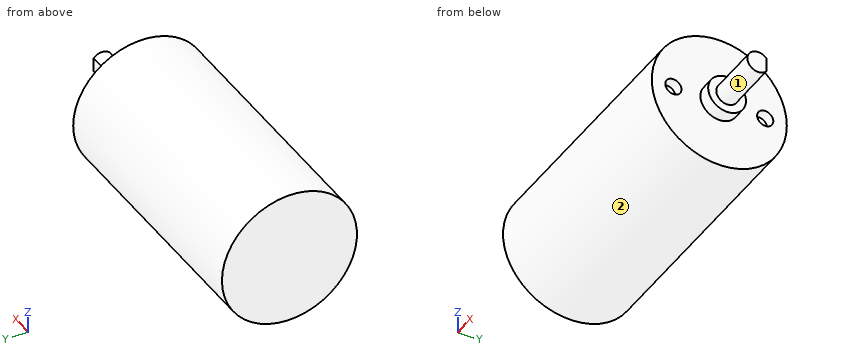
Autodesk Inventor part; units mm, degrees
ref_plane "YZ Plane" through (0, 0, 0) normal (1, 0, 0) x (0, 1, 0)
ref_plane "XZ Plane" through (0, 0, 0) normal (0, 1, 0) x (-1, 0, 0)
ref_plane "XY Plane" through (0, 0, 0) normal (0, 0, 1) x (1, 0, 0)
sketch "Sketch1" plane through (0, 0, 0) normal (1, 0, 0) x (0, 1, 0)
  circle A0 centre (0, 0) radius 12.5
  dimension "d0" = 25
extrude "Extrusion1" add sketch "Sketch1" along normal blind 47.8
sketch "Sketch2" plane through (47.8, 0, 0) normal (1, 0, 0) x (0, 0, -1)
  circle A0 centre (0, -8.5) radius 1.5
  circle A1 centre (0, 8.5) radius 1.5
  circle A2 centre (0, 0) radius 3.5
  dimension "d4" = 3
  dimension "d5" = 7
extrude "Extrusion2" add sketch "Sketch2" along normal blind 2.5 contours A2
extrude "Extrusion3" cut sketch "Sketch2" against normal blind 2 contours A0 | A1
sketch "Sketch3" plane through (50.3, 0, 0) normal (1, 0, 0) x (0, 0, -1)
  circle A0 centre (0, 0) radius 2
  dimension "d10" = 4
extrude "Extrusion4" add sketch "Sketch3" along normal blind 10
sketch "Sketch4" plane through (60.3, 0, 0) normal (1, 0, 0) x (0, 0, -1)
  circle A0 centre (0, 0) radius 2
  line L0 (0, -2) -> (0, 1.5)
  line L1 (0, 1.5) -> (1.3229, 1.5)
  line L2 (-1.3229, 1.5) -> (0, 1.5)
  arc A1 (1.3229, 1.5) -> (-1.3229, 1.5) centre (0, 0) ccw
  dimension "d13" = 3.5
extrude "Extrusion5" cut sketch "Sketch4" against normal blind 8 contours L1 L2 A0
properties part number "small motor"
Part model, mm, in its own coordinate system. Face numbers are marked on the shaded views. A direction names the side the tool comes from. Give positions to 0.01 mm unless a question says otherwise; leave off trailing zeros. Order: outer loops, then holes, each group sorted by start corner. A loop starts at its lowest first (then second) coordinate and runs counter-clockwise, first axis right, second up. Notation, with made-up numbers: (74.25, 11) - (125.25, 11) arc R12 ccw to (125.25, 19) - close; hole circle Ø8 at (38, 79). An arc over 180 degrees is marked (long way). Use a Markdown table: item, result.
1) Probe L1, parallel to X at y = 7.75, z = 9.75; L2, parallel to Y at x = 45.5, z = -0.5; L3, parallel to Z at x = 21.5, y = 8. List the from-to ranges inside material, lowest first. Write a range as from..to.
Checked values:
| item | result |
|---|---|
| L1 | 0..47.8 |
| L2 | -12.49..12.49 |
| L3 | -9.6..9.6 |
2) Flat gauge pins, fed straight in: P1, Ø8, axis at x = 29, y = -8, coming from the +Z side; P2, Ø1.5, axis at x = 13.5, y = -9.5, coming from the -Z side; P3, Ø0.9, axis at y = 9, z = 0, coming from the +X side. Where does each tip first touch, or does it go through?
Checked values:
| item | result |
|---|---|
| P1 | z = 11.84 |
| P2 | z = -8.93 |
| P3 | x = 45.8 |
3) Saw through at D-D on y = 8.5. List the corners of the cut face in (x, z).
Checked values:
| item | result |
|---|---|
| outline | (0, -9.17) - (47.8, -9.17) - (47.8, -1.5) - (45.8, -1.5) - (45.8, 1.5) - (47.8, 1.5) - (47.8, 9.17) - (0, 9.17) - close |
4) Saw through at A-A on y = 0. List the corners of the cut face in (x, z), plus the area to 3 significant figures.
Checked values:
| item | result |
|---|---|
| outline | (0, -12.5) - (47.8, -12.5) - (47.8, -3.5) - (50.3, -3.5) - (50.3, -2) - (60.3, -2) - (60.3, 2) - (50.3, 2) - (50.3, 3.5) - (47.8, 3.5) - (47.8, 12.5) - (0, 12.5) - close |
| area | 1,250 mm² |
5) 3-axis set-ups, long thin cutter, end or side, ignore diameter. For the marked faces 1 and 2: which of +Z, -Z, +X, -X, +Y, -Y reach the whole face in a straight line?
Checked values:
| item | result |
|---|---|
| face 1 | +X |
| face 2 | +X, -X |
6) Saw through at C-C on x = 12.5. List the corners of the cut face in (y, z).
Checked values:
| item | result |
|---|---|
| outline | circle Ø25 at (0, 0) |
7) Saw through at B-B on z = 0. List the corners of the cut face in (x, y).
Checked values:
| item | result |
|---|---|
| outline | (0, -12.5) - (47.8, -12.5) - (47.8, -10) - (45.8, -10) - (45.8, -7) - (47.8, -7) - (47.8, -3.5) - (50.3, -3.5) - (50.3, -2) - (60.3, -2) - (60.3, 1.5) - (52.3, 1.5) - (52.3, 2) - (50.3, 2) - (50.3, 3.5) - (47.8, 3.5) - (47.8, 7) - (45.8, 7) - (45.8, 10) - (47.8, 10) - (47.8, 12.5) - (0, 12.5) - close |
